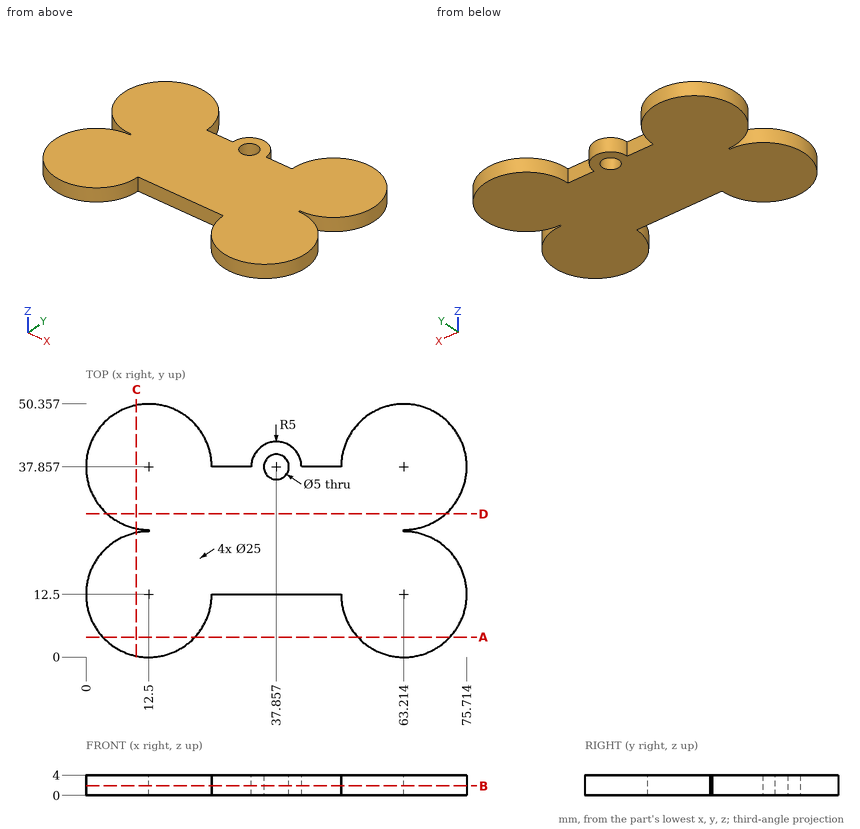
Job drawing, mm, ordinate dimensions from the low corner. One solid piece. Coordinates: 2 decimals unless noted, no trailing zeros. Write each loop counter-clockwise with the first axis right and the second up, starting at its lowest first coordinate (ties: lowest second). Pieces come first, ordered by that corner, then holes. Notation, with made-up numbers: (-16.5, -39.5) - (4.5, -39.5) arc R12 cw to (4.5, -22.5) - close; hole circle Ø11 at (71, 33). An arc over 180 degrees is marked (long way). Use a Markdown table: item, result. Add a question column.
Item 1: Drill centre lines: L1, parallel to Y at x = 47, z = 0.2; L2, parallel to X at y = 10, z = 2.2; L3, parallel to Y at x = 10.5, z = 3.2. Where is each one in solid material? Low to high. Write a range as from..to.
Item 2: Band-saw the part on A-A, the plane y = 4. Give the cut face in (x, z).
Item 3: Flat gauge pins, fed straight in: pin 1 (2 mm diameter, centred on x = 51, z = 2, fed in from +Y); pin 2 (1 mm diameter, centred on x = 42, z = 3, fed in from +Y); pin 3 (2 mm diameter, centred on y = 42, z = 2, fed in from -X). Where does each tip first touch, or does it go through?
Item 4: Band-saw the part on B-B, the plane z = 1.9. Give the cut face in (x, y).
Item 5: Band-saw the part on D-D, the plane y = 28.5. Give the cut face in (x, z).
Item 6: Band-saw the part on C-C, the plane x = 10. Give the cut face in (y, z).
Numbers:
| question | item | result |
|---|---|---|
| 1 | L1 | 12.5..37.86 |
| 1 | L2 | 0.25..24.75, 50.97..75.46 |
| 1 | L3 | 0.16..24.84, 25.52..50.2 |
| 2 | outline | (3.33, 0) - (21.67, 0) - (21.67, 4) - (3.33, 4) - close; (54.05, 0) - (72.38, 0) - (72.38, 4) - (54.05, 4) - close |
| 3 | pin 1 | y = 43.38 |
| 3 | pin 2 | y = 41.28 |
| 3 | pin 3 | x = 0.4 |
| 4 | outline | (12.5, 25) arc R12.5 ccw (long way) to (25, 12.5) - (50.71, 12.5) arc R12.5 ccw (long way) to (63.21, 25) - (63.21, 25.36) arc R12.5 ccw (long way) to (50.71, 37.86) - (42.86, 37.86) arc R5 ccw to (32.86, 37.86) - (25, 37.86) arc R12.5 ccw (long way) to (12.5, 25.36) - close; hole circle Ø5 at (37.86, 37.86) |
| 5 | outline | (4.21, 0) - (71.5, 0) - (71.5, 4) - (4.21, 4) - close |
| 6 | outline | (0.25, 0) - (24.75, 0) - (24.75, 4) - (0.25, 4) - close; (25.61, 0) - (50.1, 0) - (50.1, 4) - (25.61, 4) - close |
